Source: three-view drawing plus pictorial views. Frame: mm from the lowest corner of the part. A direction names the side the tool comes from. Round coordinates to 2 decimals unless told otherwise and drop trailing zeros. Loops run counter-clockwise (first coordinate to the right, second up) from the corner with the lowest first, then second, coordinate; pieces in that order, holes last. Notation, with made-up numbers: (22.25, 77.5) -> (80.25, 77.5) arc R26 cw to (80.25, 97.5) -> close; hole circle Ø10 at (8, 71). An arc over 180 degrees is marked (long way). One line per question, with ' | ' between items. Start each with the question number.
Q1. Cut plane D-D on x = 22. Return loops of the section in (y, z), and give its area (3 significant figures).
Q2. Contact query for flat-ended pins moving along their axis: P1, Ø1.5, axis at x = 17, y = 2, coming from the -Z side; P2, Ø1.5, axis at y = 1.5, z = 2.5, coming from the -X side; P3, Ø8, axis at x = 13, z = 7, coming from the -Y side. Output: stop coordinate, or through.
Q3. Mould query, pull axis Z, two halves, no side actions, for the marked faces 4, 5 and 6. Classes: pulls with the +Z half, pulls with the -Z half, needs draft (parallel to the pull), parting line crosses it, or undercut.
Q4. Access query for the marked faces 1, 2 and 3. Directions: +Z, -Z, +X, -X, +Y, -Y. A direction counts if a zero-diameter tool reaches every point of the face in a straight line with its end or side. Return the directions, or none.
Q5. Cut plane B-B on x = 7.5. Return loops of the section in (y, z).
Q6. Cut plane C-C on y = 1.85. Return loops of the section in (x, z), and give its area (3 significant figures).
Q7. Cut plane A-A on z = 3. Return loops of the section in (x, y).
Q8. Material intervals for L1, parallel to X at y = 2.4, z = 3.75; L2, parallel to X at y = 1.15, z = 7.75; L3, parallel to Z at x = 6.5, y = 2.85, sorted ascending.
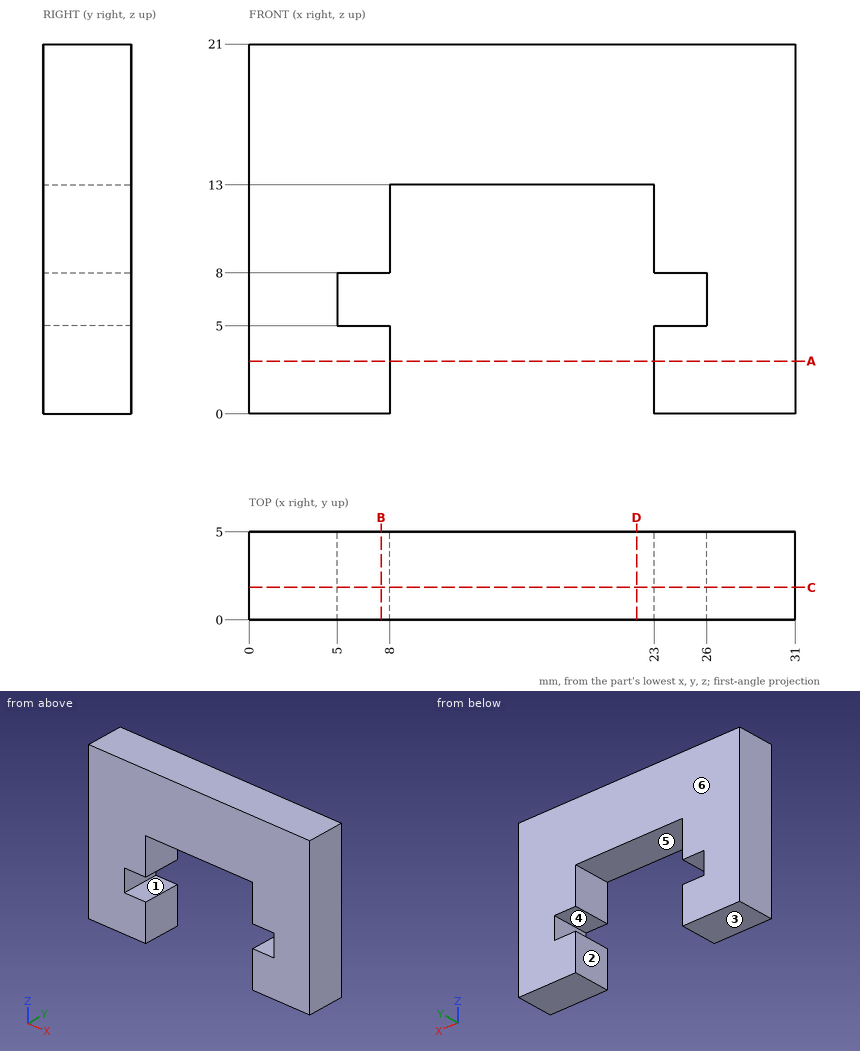
Results:
1) outline: (0, 13) -> (5, 13) -> (5, 21) -> (0, 21) -> close | area: 40.0 mm^2
2) P1: z = 13 | P2: x = 0 | P3: through
3) face 4: undercut | face 5: pulls with the -Z half | face 6: needs draft
4) face 1: +Y, -Y | face 2: -Z, +Y, -Y | face 3: -Z, +X, -X, +Y, -Y
5) outline: (0, 0) -> (5, 0) -> (5, 5) -> (0, 5) -> close; (0, 8) -> (5, 8) -> (5, 21) -> (0, 21) -> close
6) outline: (0, 0) -> (8, 0) -> (8, 5) -> (5, 5) -> (5, 8) -> (8, 8) -> (8, 13) -> (23, 13) -> (23, 8) -> (26, 8) -> (26, 5) -> (23, 5) -> (23, 0) -> (31, 0) -> (31, 21) -> (0, 21) -> close | area: 438 mm^2
7) outline: (0, 0) -> (8, 0) -> (8, 5) -> (0, 5) -> close; (23, 0) -> (31, 0) -> (31, 5) -> (23, 5) -> close
8) L1: 0 to 8, 23 to 31 | L2: 0 to 5, 26 to 31 | L3: 0 to 5, 8 to 21
